from build123d import *

# Parameters (mm, degrees)
SKETCH1_R                = 10
BOSS_EXTRUDE1_DEPTH      = 6.35
M3_CLEARANCE_HOLE1_D     = 3.4
M3_CLEARANCE_HOLE3_D     = 3.4
M3_CLEARANCE_HOLE3_DEPTH = 7
M3_CLEARANCE_HOLE3_TIP   = 1.021463052
FILLET1_R                = 1


with BuildPart() as part:
    # Sketch1 → Boss-Extrude1 (new body)
    with BuildSketch(Plane(origin=(0, 0, 0), x_dir=(1, 0, 0), z_dir=(0, 1, 0))):
        with BuildLine():
            Line((33.34, 50), (33.34, -50))
            Line((33.34, -50), (25.84, -50))
            Line((25.84, -50), (25.84, -42.5))
            ThreePointArc((25.84, -42.5), (17.131517738, -26.413305851), (0, -20))
            ThreePointArc((0, -20), (-20, 0), (0, 20))
            ThreePointArc((0, 20), (17.131517738, 26.413305851), (25.84, 42.5))
            Line((25.84, 42.5), (25.84, 50))
            Line((25.84, 50), (33.34, 50))
        make_face()
        with Locations(Location((0, 0, 0), (0, 0, 270))):
            Circle(SKETCH1_R, mode=Mode.SUBTRACT)
    extrude(amount=BOSS_EXTRUDE1_DEPTH)

    # M3 Clearance Hole1 (through all)
    with Locations(Plane(origin=(0, 6.35, 0), x_dir=(1, 0, 0), z_dir=(0, 1, 0))):
        with Locations((0, 15), (12.991881057, -7.499133975), (-12.988881057, -7.500866025), (0.001, 0)):
            Hole(M3_CLEARANCE_HOLE1_D / 2)

    # M3 Clearance Hole3
    with Locations(Plane(origin=(33.34, 0, 0), x_dir=(0, 0, -1), z_dir=(1, 0, 0))):
        with Locations((32.5, 3.175), (-32.5, 3.175)):
            Hole(M3_CLEARANCE_HOLE3_D / 2, depth=M3_CLEARANCE_HOLE3_DEPTH)
            with Locations((0, 0, -(M3_CLEARANCE_HOLE3_DEPTH + M3_CLEARANCE_HOLE3_TIP / 2))):  # 118° drill point
                Cone(0, M3_CLEARANCE_HOLE3_D / 2, M3_CLEARANCE_HOLE3_TIP, mode=Mode.SUBTRACT)

    # Fillet1
    fillet1_edges = [part.edges().sort_by_distance(p)[0] for p in [
        (29.59, 6.35, 50),
        (29.59, 6.35, -50),
        (29.59, 0, -50),
        (29.59, 0, 50),
    ]]
    fillet(fillet1_edges, radius=FILLET1_R)


solid = part.part
Source: CAD feature listing. Evaluate the final solid. Frame: model axes, mm. A direction names the side the tool comes from. Coordinates: 2 decimals unless noted, no trailing zeros. Order: outer loops, then holes, each group sorted by start corner. A loop starts at its lowest first (then second) coordinate and runs counter-clockwise, first axis right, second up.
Item 1: Material intervals for line 1 (Y direction, x = 30.25, z = 32.5) (3 decimals); line 2 (X direction, y = 3.5, z = 0); line 3 (Y direction, x = 31, z = -32), sorted ascending.
Output values:
line 1: y = 0 to 1.475, 4.875 to 6.35
line 2: x = -20 to -10, 10 to 33.34
line 3: y = 0 to 1.55, 4.8 to 6.35
Item 2: Cut plane B-B (x = 29). Return loops of the section in (y, z) (3 decimals).
Output values:
outline: (0, -49) arc R1 ccw to (1, -50) - (5.35, -50) arc R1 ccw to (6.35, -49) - (6.35, 49) arc R1 ccw to (5.35, 50) - (1, 50) arc R1 ccw to (0, 49) - close; hole circle Ø3.4 at (3.175, -32.5); hole circle Ø3.4 at (3.175, 32.5)
Item 3: Cut plane A-A (z = 0). Return loops of the section in (x, y), plus the area to 3 significant figures.
Output values:
outline: (-20, 0) - (-10, 0) - (-10, 6.35) - (-20, 6.35) - close; (10, 0) - (33.34, 0) - (33.34, 6.35) - (10, 6.35) - close
area: 212 mm2
Item 4: Set-up query: faces 5 (the face through (30, 3, -50)), 6 (the face through (25.84, 3, -46)), 7 (the face through (25.84, 3, 46)), 8 (the face through (29.79, 2.52, 34.07)), 9 (the face through (-20, 3, 0)). Return all of +Z, -Z, +X, -X, +Y, -Y with unobstructed straight access to the full face (end or side cutting, diameter ignored); none if empty.
Output values:
face 5: -Z, +X, -X, +Y, -Y
face 6: -Z, -X, +Y, -Y
face 7: +Z, -X, +Y, -Y
face 8: +X
face 9: -X, +Y, -Y
Item 5: Pull-direction query (X, two-part tool) for faces 1 (the face through (0.37, 3.13, -13.34)), 2 (the face through (17.33, 3.13, 26.59)), 3 (the face through (25.5, 3.2, 32.8)), 4 (the face through (11.42, 3.13, 8.15)); classes: pulls with the +X half, pulls with the -X half, needs draft (parallel to the pull), parting line crosses it, or undercut.
Output values:
face 1: undercut
face 2: pulls with the -X half
face 3: pulls with the +X half
face 4: undercut
Item 6: First-contact query: P1, Ø1.9, axis at y = 2.5, z = -44.5, coming from the -X side; P2, Ø2, axis at y = 3.175, z = 32.5, coming from the +X side. Flat tips, straight axial feed; report the tip coordinate or a pass-through.
Output values:
P1: stops at x = 25.84
P2: stops at x = 25.92
Item 7: Cut plane C-C (z = -15). Return loops of the section in (x, y).
Output values:
outline: (-13.23, 0) - (-1.7, 0) - (-1.7, 6.35) - (-13.23, 6.35) - close; (1.7, 0) - (33.34, 0) - (33.34, 6.35) - (1.7, 6.35) - close
Item 8: Cut plane D-D (z = 29.5). Return loops of the section in (x, y).
Output values:
outline: (20.14, 0) - (33.34, 0) - (33.34, 6.35) - (20.14, 6.35) - close
